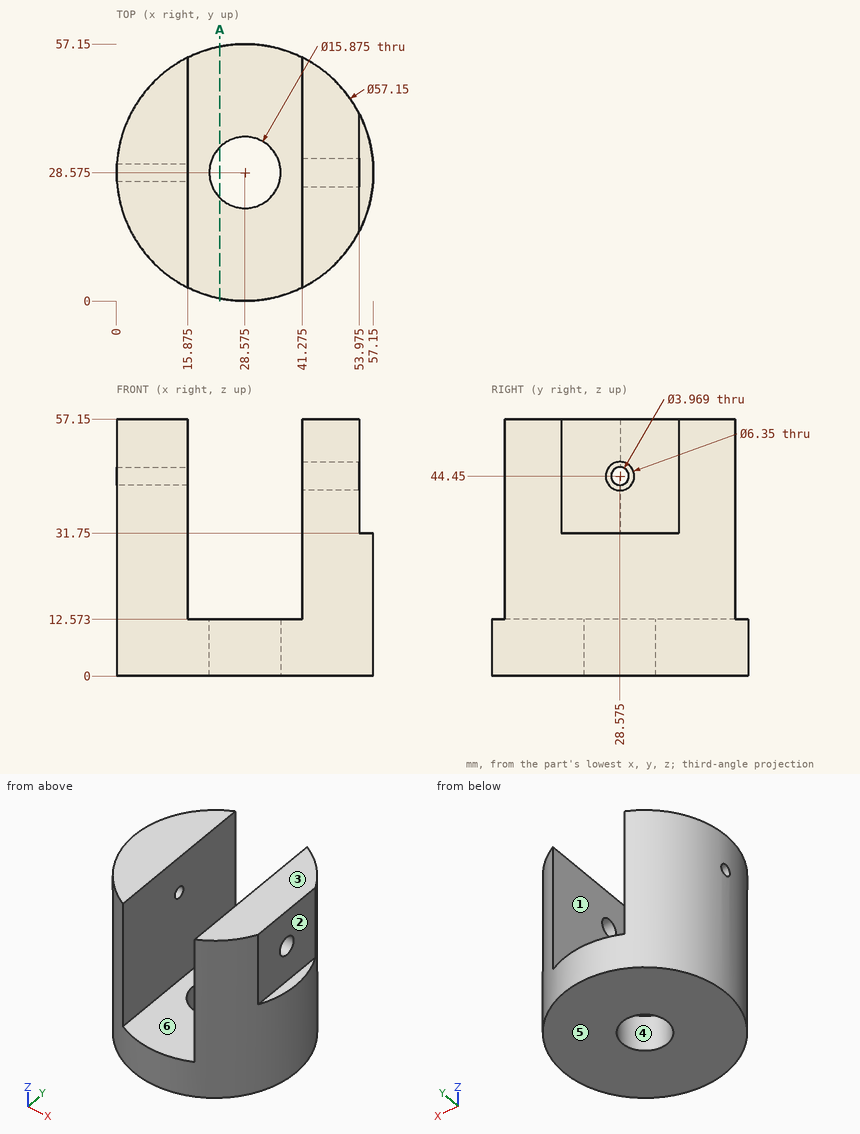
Design review of the part shown in the three views and the two pictorial views. Dimensions are in mm from the part's minimum x, y and z. A direction names the side the tool comes from. Give positions to 0.01 mm unless a question says otherwise; leave off trailing zeros. Loops run counter-clockwise (first coordinate to the right, second up) from the corner with the lowest first, then second, coordinate; pieces in that order, holes last. Notation, with made-up numbers: (-11, 51.25) -> (36, 51.25) arc R11 ccw to (36, 64.25) -> close; hole circle Ø5 at (-33, 70.5). An arc over 180 degrees is marked (long way). Answer as a JSON object with one key per item and string values. Group by question number.
Q1. Draft analysis for pull direction X (two halves, no side actions). For the marked faces 1, 2, 3 and 4, state which applies: pulls with the +X half, pulls with the -X half, needs draft (parallel to the pull), parting line crosses it, or undercut.
Q2. Insertion check: pin 1 (12 mm diameter, centred on y = 38, z = 16.5, fed in from -X); pin 2 (8 mm diameter, centred on y = 42.5, z = 29, fed in from +X); pin 3 (4 mm diameter, centred on y = 29, z = 37, fed in from +X) (3 decimals); pin 4 (2 mm diameter, centred on x = 18.5, z = 23.5, fed in from +Y). Each pin has a flat end and moves straight along its axis. Give the tip position at first contact, or say it passes through.
Q3. Take a section at A-A (x = 23). Write out the cut boundary in (y, z) (1 decimal), plus the area to 3 significant figures.
Q4. Tool access review of the marked faces 5 and 6: name each direction out of +Z, -Z, +X, -X, +Y, -Y from which nothing blocks a thin tool from reaching the whole face with its end or side.
Q5. Wall thickness on line 1 along Z through (x, y) = (36.5, 15); line 2 along X through (y, z) = (10, 37) (1 decimal); line 3 along X through (y, z) = (16, 24) (1 decimal): over which ranges is each line inside the solid? List them lowest first.
Answer below:
{
 "1": {"face 1": "undercut", "face 2": "pulls with the +X half", "face 3": "needs draft", "face 4": "undercut"},
 "2": {"pin 1": "stops at x = 0.21", "pin 2": "stops at x = 55.37", "pin 3": "stops at x = 53.975", "pin 4": "passes through"},
 "3": {"outline": "(0.5, 0) -> (22.9, 0) -> (22.9, 12.6) -> (0.5, 12.6) -> close; (34.2, 0) -> (56.6, 0) -> (56.6, 12.6) -> (34.2, 12.6) -> close", "area": "563 mm2"},
 "4": {"face 5": "-Z, +X, -X, +Y, -Y", "face 6": "+Z, +Y, -Y"},
 "5": {"line 1": "z = 0 to 12.57", "line 2": "x = 6.9 to 15.9, 41.3 to 50.3", "line 3": "x = 2.9 to 15.9, 41.3 to 54.2"}
}
